from build123d import *

# Parameters (mm, degrees)
SKETCH005_R   = 2
SKETCH005_R_2 = 2.65
PAD_DEPTH     = 4


with BuildPart() as part:
    # Sketch005 → Pad (new body)
    with BuildSketch(Plane.XY.offset(-3)):
        Polygon((-38, 10), (-9, 10), (-9, 1), (-15, 1), (-15, -1), (-9, -1), (-9, -10), (31, -10), (31, -1), (37, -1), (37, 1), (31, 1), (31, 10), (38, 10), (47, 0.7), (47, -8.030345), (28, -19), (-35, -19), (-50, -10.339746), (-50, 3.07), align=None)
        with Locations((-13.5, 5)):
            Circle(SKETCH005_R, mode=Mode.SUBTRACT)
        with Locations((-13.5, -5)):
            Circle(SKETCH005_R, mode=Mode.SUBTRACT)
        with Locations((35.5, 5)):
            Circle(SKETCH005_R, mode=Mode.SUBTRACT)
        with Locations((35.5, -5)):
            Circle(SKETCH005_R, mode=Mode.SUBTRACT)
        with Locations((-44.5, 0)):
            Circle(SKETCH005_R_2, mode=Mode.SUBTRACT)
        with Locations((40.5, -5)):
            Circle(SKETCH005_R_2, mode=Mode.SUBTRACT)
    extrude(amount=PAD_DEPTH)


solid = part.part
Could you check a few things on this model? Use its own coordinates, in mm. A direction names the side the tool comes from. Round coordinates to 2 decimals unless told otherwise and drop trailing zeros. Order: outer loops, then holes, each group sorted by start corner. A loop starts at its lowest first (then second) coordinate and runs counter-clockwise, first axis right, second up. Notation, with made-up numbers: M 14,79.5 L 28,79.5 A16 ccw 28,90.5 Z; hole C 17.5,34 d5. An arc over 180 degrees is marked long. One line per item, written item: value.
(1) Imagine slicing it at A-A (z = -2). Write out the boundary of the cut face in (x, y), and give its area (3 significant figures).
Ans:
outline: M -50,-10.34 L -35,-19 L 28,-19 L 47,-8.03 L 47,0.7 L 38,10 L 31,10 L 31,1 L 37,1 L 37,-1 L 31,-1 L 31,-10 L -9,-10 L -9,-1 L -15,-1 L -15,1 L -9,1 L -9,10 L -38,10 L -50,3.07 Z; hole C -44.5,0 d5.3; hole C -13.5,-5 d4; hole C -13.5,5 d4; hole C 35.5,-5 d4; hole C 35.5,5 d4; hole C 40.5,-5 d5.3
area: 1,640 mm^2
(2) I need wall thicknesses on line 1 along X through (y, z) = (1.25, -0.5); line 2 along X through (y, z) = (-3.75, 0.8); line 3 along X through (y, z) = (-3.5, 0.2). Which ranges of each line are inside material? Lowest first, please. Write a range as from..to.
Ans:
line 1: x = -50..-46.84, -42.16..-9, 31..46.47
line 2: x = -50..-15.06, -11.94..-9, 31..33.94, 37.06..38.16, 42.84..47
line 3: x = -50..-14.82, -12.18..-9, 31..34.18, 36.82..38.32, 42.68..47
(3) Imagine slicing it at C-C (x = -13.5). Write out the boundary of the cut face in (y, z).
Ans:
outline: M -19,-3 L -7,-3 L -7,1 L -19,1 Z; M -3,-3 L -1,-3 L -1,1 L -3,1 Z; M 1,-3 L 3,-3 L 3,1 L 1,1 Z; M 7,-3 L 10,-3 L 10,1 L 7,1 Z
(4) Which directions (+Z, -Z, +X, -X, +Y, -Y) give clear straight access to the entire face, cutting with the end or side of a thin tool? Please do faces 4 (the flat face through (11, -10, -1)), 5 (the flat face through (34, 10, -1)), 6 (the flat face through (34, 1, -1)).
Ans:
face 4: +Z, -Z, +Y
face 5: +Z, -Z, +X, -X, +Y
face 6: +Z, -Z
(5) Imagine slicing it at B-B (y = 5). Write out the boundary of the cut face in (x, z).
Ans:
outline: M -46.66,-3 L -15.5,-3 L -15.5,1 L -46.66,1 Z; M -11.5,-3 L -9,-3 L -9,1 L -11.5,1 Z; M 31,-3 L 33.5,-3 L 33.5,1 L 31,1 Z; M 37.5,-3 L 42.84,-3 L 42.84,1 L 37.5,1 Z
(6) I'm going to push flat-ended pins straight in: P1, Ø4.5, axis at x = -13.5, y = 5, coming from the -Z side; P2, Ø1.2, axis at x = 7, z = -1.5, coming from the +Y side; P3, Ø2, axis at x = 34, z = -1, coming from the -Y side. Where does each tip first touch, or does it pass through?
Ans:
P1: stops at z = -3
P2: stops at y = -10
P3: stops at y = -16.11
(7) Imagine slicing it at D-D (x = 40.5). Write out the boundary of the cut face in (y, z), and give its area (3 significant figures).
Ans:
outline: M -11.78,-3 L -7.65,-3 L -7.65,1 L -11.78,1 Z; M -2.35,-3 L 7.42,-3 L 7.42,1 L -2.35,1 Z
area: 55.6 mm^2
(8) If we mould it in two halves opening along Y, with no side actions, what happens to faces 1 (the cylindrical face through (-15.498, 5.088, -1.028)), 2 (the flat face through (47, -4, -1)), 3 (the flat face through (-44.08, 6.49, -1.03))? For each: released by +Y, released by -Y, zero draft, split by the parting line, or undercut.
Ans:
face 1: undercut
face 2: zero draft
face 3: released by +Y
